Design review of the part built by this model. Coordinates are the model's own, in mm. Face numbers are marked on the shaded views. A direction names the side the tool comes from. Give positions to 0.01 mm unless a question says otherwise; leave off trailing zeros. Write each loop counter-clockwise with the first axis right and the second up, starting at its lowest first coordinate (ties: lowest second). Pieces come first, ordered by that corner, then holes.
```python
from build123d import *

# Parameters (mm, degrees)
SKETCH1_W           = 63.5
SKETCH1_H           = 48.26
BOSS_EXTRUDE1_DEPTH = 55.626
SKETCH2_W           = 31.75
SKETCH2_H           = 19.05
SKETCH2_W_2         = 15.242568483
SKETCH2_H_2         = 31.496
SKETCH2_W_3         = 6.35
SKETCH2_H_3         = 16.256
SKETCH2_W_4         = 15.875
CUT_EXTRUDE2_DEPTH  = 64.5
SKETCH3_W           = 23.876
SKETCH3_H           = 36.576
SKETCH3_W_2         = 14.224
CUT_EXTRUDE3_DEPTH  = 49.26
SKETCH4_R           = 1.27
CUT_EXTRUDE4_DEPTH  = 33.385
CUT_EXTRUDE6_REACH  = 50.26
SKETCH6_R           = 3.302
SKETCH7_R           = 3.302
CUT_EXTRUDE7_DEPTH  = 49.26
CUT_EXTRUDE11_DEPTH = 11.43
SKETCH10_R          = 0.889
CUT_EXTRUDE10_DEPTH = 6.35
SKETCH9_R           = 0.889
CUT_EXTRUDE9_DEPTH  = 6.35


with BuildPart() as part:
    # Sketch1 → Boss-Extrude1 (new body)
    with BuildSketch(Plane(origin=(0, 0, 0), x_dir=(1, 0, 0), z_dir=(0, 1, 0))):
        with Locations((31.75, 24.13)):
            Rectangle(SKETCH1_W, SKETCH1_H)
    extrude(amount=BOSS_EXTRUDE1_DEPTH)

    # Sketch2 → Cut-Extrude2 (cut, through all)
    with BuildSketch(Plane(origin=(63.5, 0, 0), x_dir=(0, 0, -1), z_dir=(1, 0, 0))):
        with Locations((24.765, 9.525)):
            Rectangle(SKETCH2_W, SKETCH2_H)
        with Locations((40.638715758, 39.878)):
            Rectangle(SKETCH2_W_2, SKETCH2_H_2)
        with Locations((24.13, 47.498)):
            Rectangle(SKETCH2_W_3, SKETCH2_H_3)
        with Locations((7.9375, 39.878)):
            Rectangle(SKETCH2_W_4, SKETCH2_H_2)
    extrude(amount=-CUT_EXTRUDE2_DEPTH, mode=Mode.SUBTRACT)

    # Sketch3 → Cut-Extrude3 (cut, through all)
    with BuildSketch(Plane.XY):
        with Locations((11.938, 37.338)):
            Rectangle(SKETCH3_W, SKETCH3_H)
        with Locations((56.388, 37.338)):
            Rectangle(SKETCH3_W_2, SKETCH3_H)
    extrude(amount=-CUT_EXTRUDE3_DEPTH, mode=Mode.SUBTRACT)

    # Sketch4 → Cut-Extrude4 (cut, through all)
    with BuildSketch(Plane.XY.offset(-15.875)):
        with Locations((36.576, 53.086)):
            Circle(SKETCH4_R)
    extrude(amount=-CUT_EXTRUDE4_DEPTH, mode=Mode.SUBTRACT)

    # Sketch6 → Cut-Extrude6 (cut, up to next)
    with BuildSketch(Plane(origin=(0, 0, -48.26), x_dir=(-1, 0, 0), z_dir=(0, 0, -1)), mode=Mode.PRIVATE) as cut_extrude6_sk1:
        with Locations((-15.24, 12.7)):
            Circle(SKETCH6_R)
    cut_extrude6_tool1 = extrude(cut_extrude6_sk1.sketch, amount=-CUT_EXTRUDE6_REACH, mode=Mode.PRIVATE) & part.part
    add(cut_extrude6_tool1.solids().sort_by_distance((15.24, 12.7, -48.26))[0], mode=Mode.SUBTRACT)

    # Sketch7 → Cut-Extrude7 (cut, through all)
    with BuildSketch(Plane(origin=(0, 0, -48.26), x_dir=(-1, 0, 0), z_dir=(0, 0, -1))):
        with Locations((-15.24, 12.7)):
            Circle(SKETCH7_R)
    extrude(amount=-CUT_EXTRUDE7_DEPTH, mode=Mode.SUBTRACT)

    # Sketch8 → Cut-Extrude11 (cut)
    with BuildSketch(Plane(origin=(0, 0, -48.26), x_dir=(-1, 0, 0), z_dir=(0, 0, -1))):
        with BuildLine():
            Line((-49.276, 24.13), (-46.013321356, 24.13))
            Line((-46.013321356, 24.13), (-46.013321356, 11.43))
            ThreePointArc((-46.013321356, 11.43), (-52.617321356, 4.826), (-59.221321356, 11.43))
            Line((-59.221321356, 11.43), (-59.221321356, 19.05))
            Line((-59.221321356, 19.05), (-49.276, 19.05))
            Line((-49.276, 19.05), (-49.276, 24.13))
        make_face()
    extrude(amount=-CUT_EXTRUDE11_DEPTH, mode=Mode.SUBTRACT)

    # Sketch10 → Cut-Extrude10 (cut)
    with BuildSketch(Plane(origin=(63.5, 0, 0), x_dir=(0, 0, -1), z_dir=(1, 0, 0))):
        with Locations((6.26745, 11.43)):
            Circle(SKETCH10_R)
        with Locations((44.13885, 11.43)):
            Circle(SKETCH10_R)
    extrude(amount=-CUT_EXTRUDE10_DEPTH, mode=Mode.SUBTRACT)

    # Sketch9 → Cut-Extrude9 (cut)
    with BuildSketch(Plane(origin=(63.5, 0, 0), x_dir=(0, 0, -1), z_dir=(1, 0, 0))):
        with Locations((5.969, 11.303)):
            Circle(SKETCH9_R)
        with Locations((43.815, 11.303)):
            Circle(SKETCH9_R)
    extrude(amount=-CUT_EXTRUDE9_DEPTH, mode=Mode.SUBTRACT)


solid = part.part
```
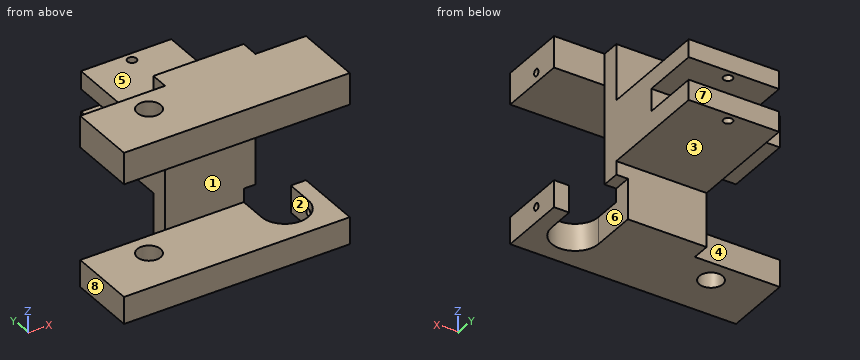
(1) Clearance check with flat-ended pins moving along their axes: P1, Ø7.5, axis at x = 32.5, y = 42, coming from the +Z side (3 decimals); P2, Ø12, axis at x = 43.5, y = 35, coming from the -Z side; P3, Ø4.5, axis at x = 53.5, z = -3, coming from the +Y side. State where each tip first meets the part, or that it passes through.
Resolved:
P1: stops at z = -15.875
P2: stops at z = -33.02
P3: stops at y = 19.05
(2) Consider section D-D, the plane z = -39. Give the boundary of the cut face in (x, y), then the cut area to 3 significant figures.
Resolved:
outline: (23.88, 19.05) - (46.01, 19.05) - (46.01, 24.13) - (23.88, 24.13) - close
area: 112 mm2
(3) Tool access review of the marked faces 1, 2, 3, 4 and 5: name each direction out of +Z, -Z, +X, -X, +Y, -Y from which nothing blocks a thin tool from reaching the whole face with its end or side.
Resolved:
face 1: +X, -X, -Y
face 2: -Z, +Y
face 3: -Z, +X, -X, +Y
face 4: +Z, -Z, -X, +Y
face 5: +Z, +X, -X, +Y
(4) Consider section A-A, the plane x = 15.24. Give the boundary of the cut face in (y, z), then the cut area to 3 significant figures.
Resolved:
outline: (0, -48.26) - (9.4, -48.26) - (9.4, -40.64) - (0, -40.64) - close; (0, -8.89) - (9.4, -8.89) - (9.4, 0) - (0, 0) - close; (16, -48.26) - (19.05, -48.26) - (19.05, -40.64) - (16, -40.64) - close; (16, -8.89) - (19.05, -8.89) - (19.05, 0) - (16, 0) - close
area: 205 mm2
(5) Mouldability with a two-part tool opening along X and no side actions: class the marked faces 6, 7 and 8 as pulls with the +X half, pulls with the -X half, needs draft (parallel to the pull), parting line crosses it, or undercut.
Resolved:
face 6: undercut
face 7: needs draft
face 8: pulls with the -X half
(6) Consider section B-B, the plane y = 49. Give the boundary of the cut face in (x, z) (3 decimals).
Resolved:
outline: (23.876, -33.017) - (49.276, -33.017) - (49.276, -27.305) - (23.876, -27.305) - close; (23.876, -20.955) - (49.276, -20.955) - (49.276, -15.875) - (23.876, -15.875) - close
(7) Consider section C-C, the plane y = 8.5. Give the boundary of the cut face in (x, z).
Resolved:
outline: (0, -48.26) - (46.7, -48.26) - (46.7, -40.64) - (0, -40.64) - close; (0, -8.89) - (63.5, -8.89) - (63.5, 0) - (0, 0) - close; (58.54, -48.26) - (63.5, -48.26) - (63.5, -40.64) - (58.54, -40.64) - close
(8) To check wall thickness, follow L1, parallel to Z at x = 61.5, y = 11.43; L2, parallel to Z at x = 61.5, y = 7; L3, parallel to Z at x = 24.5, y = 42 (3 decimals). State the ranges of each line that lie inside material, in increasing order.
Resolved:
L1: z = -48.26 to -45.03, -42.94 to -40.64, -8.89 to -7.16, -5.09 to 0
L2: z = -48.26 to -40.64, -8.89 to 0
L3: z = -33.017 to -27.305, -20.955 to -15.875
